Model file for the job. Use its own axes, mm. A direction names the side the tool comes from. Coordinates: 2 decimals unless noted, no trailing zeros. Write each loop counter-clockwise with the first axis right and the second up, starting at its lowest first coordinate (ties: lowest second). Pieces come first, ordered by that corner, then holes. Notation, with made-up numbers: M 27,89 L 68,89 A19 cw 68,110 Z; hole C -6,35.25 d11. An arc over 180 degrees is marked long. One line per question, with ' | ' between items. Start each with the question number.
(1) Cut at A-A (z = 7). Write the cut outline in (x, y) (1 decimal), plus the area to 3 significant figures.
(2) Two-plate mould, pull along X, no slides. Class faces 1 (the face through (-3.1, -0.69, -30.31)), 2 (the face through (-1, -1, 28.575)), 3 (the face through (-0.043, -0.192, 20.394)): +X half, -X half, draft (parallel to the pull), parting line (faces both ways), or undercut.
(3) Wall check: probe 1 along X at (y, z) = (0, 24.25); probe 2 along Z at (x, y) = (2, 0) (3 decimals); probe 3 along Y at (x, z) = (0.5, 23). Give the ranges that are in metal, low to high.
(4) Flat gauge pins, fed straight in: pin 1 Ø1 at (x, z) = (0, 3) entering from -Y; pin 2 Ø3 at (y, z) = (2, 7) entering from +X. Where does each tip first touch, or does it go through?
(5) Tool access for faces 4 (the face through (0, 0, -31.75)), 5 (the face through (0.245, -1.103, 24.712)): list every direction of +Z, -Z, +X, -X, +Y, -Y with a clear straight run to the whole face (end or side of a thin tool).
from build123d import *

# Parameters (mm, degrees)
SKETCH1_W                 = 57.15
SKETCH1_H                 = 1.5875
F_4_40_TAPPED_HOLE1_D     = 2.2606
F_4_40_TAPPED_HOLE1_DEPTH = 7.62
F_4_40_TAPPED_HOLE1_TIP   = 0.679152758


with BuildPart() as part:
    # Sketch1 → Revolve1 (revolve)
    with BuildSketch(Plane(origin=(0, 0, 0), x_dir=(0, 0, -1), z_dir=(1, 0, 0))):
        with Locations((0, 0.79375)):
            Rectangle(SKETCH1_W, SKETCH1_H)
        Polygon((31.75, 0), (28.575, 0), (28.575, 1.5875), (28.575, 2.1828125), (28.829, 2.1828125), (28.829, 3.175), (31.75, 3.175), align=None)
    revolve(axis=Axis((0, 0, 28.575), (0, 0, -1)))

    # #4-40 Tapped Hole1
    with Locations(Plane.XY.offset(28.575)):
        with Locations((0, 0)):
            Hole(F_4_40_TAPPED_HOLE1_D / 2, depth=F_4_40_TAPPED_HOLE1_DEPTH)
            with Locations((0, 0, -(F_4_40_TAPPED_HOLE1_DEPTH + F_4_40_TAPPED_HOLE1_TIP / 2))):  # 118° drill point
                Cone(0, F_4_40_TAPPED_HOLE1_D / 2, F_4_40_TAPPED_HOLE1_TIP, mode=Mode.SUBTRACT)


solid = part.part
Filled in:
1) outline: C 0,0 d3.2 | area: 7.92 mm²
2) face 1: parting line | face 2: draft | face 3: undercut
3) probe 1: -1.59 to -1.13, 1.13 to 1.59 | probe 2: -31.75 to -28.575 | probe 3: -1.51 to -1.01, 1.01 to 1.51
4) pin 1: y = -1.59 | pin 2: x = 1.51
5) face 4: -Z, +X, -X, +Y, -Y | face 5: +Z
